Can you work these out from the model? Positions are in its coordinate system, mm. A direction names the side the tool comes from. Coordinates: 2 decimals unless noted, no trailing zeros. Loops run counter-clockwise (first coordinate to the right, second up) from the corner with the lowest first, then second, coordinate; pieces in that order, holes last.
```python
from build123d import *
from build123d import SkipClean  # not in build123d's __all__

# Parameters (mm, degrees)
F1_DEPTH = 4
F2_DEPTH = 2


with BuildPart() as f1:
    # F0 (on Top) → F1 (new body)
    with BuildSketch(Plane.XY):
        Polygon((0, -51.35), (-3.5355339059, -54.8855339059), (54.8855339059, -54.8855339059), (51.35, -51.35), (48.35, -51.35), (44.35, -51.35), (7, -51.35), (3, -51.35), align=None)
        Polygon((7, -7), (0, -7), (0, -44.35), (7, -44.35), (7, -41.3499993608), (7, -10), align=None)
        Polygon((10.0000006392, -44.35), (7, -44.35), (7, -51.35), (44.35, -51.35), (44.35, -44.35), (41.35, -44.35), align=None)
        with BuildLine():
            Line((7, -44.35), (0, -44.35))
            Line((0, -44.35), (0, -48.35))
            Line((0, -48.35), (1.5, -48.35))
            ThreePointArc((1.5, -48.35), (3, -46.85), (4.5, -48.35))
            ThreePointArc((4.5, -48.35), (4.0606601718, -49.4106601718), (3, -49.85))
            Line((3, -49.85), (3, -51.35))
            Line((3, -51.35), (7, -51.35))
            Line((7, -51.35), (7, -44.35))
        make_face()
        with BuildLine():
            Line((0, -48.35), (0, -51.35))
            Line((0, -51.35), (3, -51.35))
            Line((3, -51.35), (3, -49.85))
            ThreePointArc((3, -49.85), (1.9393398282, -49.4106601718), (1.5, -48.35))
            Line((1.5, -48.35), (0, -48.35))
        make_face()
        Polygon((0, -3), (0, 0), (-3.5355339059, 3.5355339059), (-3.5355339059, -54.8855339059), (0, -51.35), (0, -48.35), (0, -44.35), (0, -7), align=None)
        with BuildLine():
            Line((7, 0), (3, 0))
            Line((3, 0), (3, -1.5))
            ThreePointArc((3, -1.5), (4.0606601718, -1.9393398282), (4.5, -3))
            ThreePointArc((4.5, -3), (3, -4.5), (1.5, -3))
            Line((1.5, -3), (0, -3))
            Line((0, -3), (0, -7))
            Line((0, -7), (7, -7))
            Line((7, -7), (7, 0))
        make_face()
        with BuildLine():
            Line((3, 0), (0, 0))
            Line((0, 0), (1.9393398282, -1.9393398282))
            ThreePointArc((1.9393398282, -1.9393398282), (2.4259748515, -1.6141807012), (3, -1.5))
            Line((3, -1.5), (3, 0))
        make_face()
        with BuildLine():
            Line((1.9393398282, -1.9393398282), (0, 0))
            Line((0, 0), (0, -3))
            Line((0, -3), (1.5, -3))
            ThreePointArc((1.5, -3), (1.6141807012, -2.4259748515), (1.9393398282, -1.9393398282))
        make_face()
        Polygon((-3.5355339059, 3.5355339059), (0, 0), (3, 0), (7, 0), (44.35, 0), (48.35, 0), (51.35, 0), (54.8855339059, 3.5355339059), align=None)
        Polygon((44.35, 0), (7, 0), (7, -7), (10, -7), (41.3499993608, -7), (44.35, -7), align=None)
        with BuildLine():
            Line((48.35, 0), (44.35, 0))
            Line((44.35, 0), (44.35, -7))
            Line((44.35, -7), (51.35, -7))
            Line((51.35, -7), (51.35, -3))
            Line((51.35, -3), (49.85, -3))
            ThreePointArc((49.85, -3), (47.2893398282, -4.0606601718), (48.35, -1.5))
            Line((48.35, -1.5), (48.35, 0))
        make_face()
        with BuildLine():
            Line((51.35, -3), (51.35, 0))
            Line((51.35, 0), (48.35, 0))
            Line((48.35, 0), (48.35, -1.5))
            ThreePointArc((48.35, -1.5), (49.4106601718, -1.9393398282), (49.85, -3))
            Line((49.85, -3), (51.35, -3))
        make_face()
        Polygon((54.8855339059, -54.8855339059), (54.8855339059, 3.5355339059), (51.35, 0), (51.35, -3), (51.35, -7), (51.35, -44.35), (51.35, -48.35), (51.35, -51.35), align=None)
        Polygon((51.35, -7), (44.35, -7), (44.35, -10.0000006392), (44.35, -41.35), (44.35, -44.35), (51.35, -44.35), align=None)
        with BuildLine():
            Line((48.35, -51.35), (51.35, -51.35))
            Line((51.35, -51.35), (51.35, -48.35))
            Line((51.35, -48.35), (49.85, -48.35))
            ThreePointArc((49.85, -48.35), (49.4106601718, -49.4106601718), (48.35, -49.85))
            Line((48.35, -49.85), (48.35, -51.35))
        make_face()
        with BuildLine():
            Line((44.35, -51.35), (48.35, -51.35))
            Line((48.35, -51.35), (48.35, -49.85))
            ThreePointArc((48.35, -49.85), (47.2893398282, -47.2893398282), (49.85, -48.35))
            Line((49.85, -48.35), (51.35, -48.35))
            Line((51.35, -48.35), (51.35, -44.35))
            Line((51.35, -44.35), (44.35, -44.35))
            Line((44.35, -44.35), (44.35, -51.35))
        make_face()
        Polygon((7, -41.3499993608), (7, -44.35), (8.5000003196, -42.8499996804), align=None)
        Polygon((8.5000003196, -42.8499996804), (7, -44.35), (10.0000006392, -44.35), align=None)
        Polygon((8.5000003196, -42.8499996804), (10.0000006392, -44.35), (25.6750003196, -28.6750003196), (24.175, -27.175), align=None)
        Polygon((22.6749996804, -25.6749996804), (7, -41.3499993608), (8.5000003196, -42.8499996804), (24.175, -27.175), align=None)
        Polygon((8.5, -8.5), (7, -10), (22.6749996804, -25.6749996804), (24.1749996804, -24.1749996804), align=None)
        Polygon((25.6749996804, -22.6749996804), (10, -7), (8.5, -8.5), (24.1749996804, -24.1749996804), align=None)
        Polygon((27.175, -24.175), (25.6749996804, -22.6749996804), (24.1749996804, -24.1749996804), (25.675, -25.675), align=None)
        Polygon((27.1750003196, -27.1750003196), (28.6750003196, -25.6750003196), (27.175, -24.175), (25.675, -25.675), align=None)
        Polygon((25.675, -25.675), (24.175, -27.175), (25.6750003196, -28.6750003196), (27.1750003196, -27.1750003196), align=None)
        Polygon((24.1749996804, -24.1749996804), (22.6749996804, -25.6749996804), (24.175, -27.175), (25.675, -25.675), align=None)
        Polygon((25.6750003196, -28.6750003196), (41.35, -44.35), (42.85, -42.85), (27.1750003196, -27.1750003196), align=None)
        Polygon((42.85, -42.85), (44.35, -41.35), (28.6750003196, -25.6750003196), (27.1750003196, -27.1750003196), align=None)
        Polygon((8.5, -8.5), (7, -7), (7, -10), align=None)
        Polygon((10, -7), (7, -7), (8.5, -8.5), align=None)
        Polygon((28.6750003196, -25.6750003196), (44.35, -10.0000006392), (42.8499996804, -8.5000003196), (27.175, -24.175), align=None)
        Polygon((42.8499996804, -8.5000003196), (41.3499993608, -7), (25.6749996804, -22.6749996804), (27.175, -24.175), align=None)
        Polygon((44.35, -10.0000006392), (44.35, -7), (42.8499996804, -8.5000003196), align=None)
        Polygon((44.35, -44.35), (44.35, -41.35), (42.85, -42.85), align=None)
        Polygon((42.85, -42.85), (41.35, -44.35), (44.35, -44.35), align=None)
        Polygon((42.8499996804, -8.5000003196), (44.35, -7), (41.3499993608, -7), align=None)
    extrude(amount=F1_DEPTH)

    # F0 (on Top) → F2 (join)
    with BuildSketch(Plane.XY):
        with BuildLine():
            Line((7, -44.35), (0, -44.35))
            Line((0, -44.35), (0, -48.35))
            Line((0, -48.35), (1.5, -48.35))
            ThreePointArc((1.5, -48.35), (3, -46.85), (4.5, -48.35))
            ThreePointArc((4.5, -48.35), (4.0606601718, -49.4106601718), (3, -49.85))
            Line((3, -49.85), (3, -51.35))
            Line((3, -51.35), (7, -51.35))
            Line((7, -51.35), (7, -44.35))
        make_face()
        with BuildLine():
            Line((0, -48.35), (0, -51.35))
            Line((0, -51.35), (3, -51.35))
            Line((3, -51.35), (3, -49.85))
            ThreePointArc((3, -49.85), (1.9393398282, -49.4106601718), (1.5, -48.35))
            Line((1.5, -48.35), (0, -48.35))
        make_face()
        with BuildLine():
            Line((44.35, -51.35), (48.35, -51.35))
            Line((48.35, -51.35), (48.35, -49.85))
            ThreePointArc((48.35, -49.85), (47.2893398282, -47.2893398282), (49.85, -48.35))
            Line((49.85, -48.35), (51.35, -48.35))
            Line((51.35, -48.35), (51.35, -44.35))
            Line((51.35, -44.35), (44.35, -44.35))
            Line((44.35, -44.35), (44.35, -51.35))
        make_face()
        with BuildLine():
            Line((48.35, -51.35), (51.35, -51.35))
            Line((51.35, -51.35), (51.35, -48.35))
            Line((51.35, -48.35), (49.85, -48.35))
            ThreePointArc((49.85, -48.35), (49.4106601718, -49.4106601718), (48.35, -49.85))
            Line((48.35, -49.85), (48.35, -51.35))
        make_face()
        with BuildLine():
            Line((48.35, 0), (44.35, 0))
            Line((44.35, 0), (44.35, -7))
            Line((44.35, -7), (51.35, -7))
            Line((51.35, -7), (51.35, -3))
            Line((51.35, -3), (49.85, -3))
            ThreePointArc((49.85, -3), (47.2893398282, -4.0606601718), (48.35, -1.5))
            Line((48.35, -1.5), (48.35, 0))
        make_face()
        with BuildLine():
            Line((51.35, -3), (51.35, 0))
            Line((51.35, 0), (48.35, 0))
            Line((48.35, 0), (48.35, -1.5))
            ThreePointArc((48.35, -1.5), (49.4106601718, -1.9393398282), (49.85, -3))
            Line((49.85, -3), (51.35, -3))
        make_face()
        with BuildLine():
            Line((7, 0), (3, 0))
            Line((3, 0), (3, -1.5))
            ThreePointArc((3, -1.5), (4.0606601718, -1.9393398282), (4.5, -3))
            ThreePointArc((4.5, -3), (3, -4.5), (1.5, -3))
            Line((1.5, -3), (0, -3))
            Line((0, -3), (0, -7))
            Line((0, -7), (7, -7))
            Line((7, -7), (7, 0))
        make_face()
        with BuildLine():
            Line((1.9393398282, -1.9393398282), (0, 0))
            Line((0, 0), (0, -3))
            Line((0, -3), (1.5, -3))
            ThreePointArc((1.5, -3), (1.6141807012, -2.4259748515), (1.9393398282, -1.9393398282))
        make_face()
        with BuildLine():
            Line((3, 0), (0, 0))
            Line((0, 0), (1.9393398282, -1.9393398282))
            ThreePointArc((1.9393398282, -1.9393398282), (2.4259748515, -1.6141807012), (3, -1.5))
            Line((3, -1.5), (3, 0))
        make_face()
    with SkipClean():  # cleaning this boolean's faces spoils the solid; the shape is the same uncleaned
        extrude(amount=-F2_DEPTH)


solid = f1.part
```
(1) I want a section at D-D on y = -37.5. Write out the boundary of the cut face in (x, z).
Check values:
outline: (-3.54, 0) - (7, 0) - (7, 4) - (-3.54, 4) - close; (10.85, 0) - (16.85, 0) - (16.85, 4) - (10.85, 4) - close; (34.5, 0) - (40.5, 0) - (40.5, 4) - (34.5, 4) - close; (44.35, 0) - (54.89, 0) - (54.89, 4) - (44.35, 4) - close
(2) If we mould it in two halves opening along X, with no side actions, what happens to faces 5 (the flat face through (0, -3, -1)), 6 (the flat face through (7, -48, -1)), 7 (the flat face through (26, -44.35, 2)), 8 (the flat face through (51.35, -48, -1))? For each: released by +X, released by -X, zero draft, split by the parting line, or undercut.
Check values:
face 5: released by -X
face 6: undercut
face 7: undercut
face 8: released by +X
(3) If I drill on probe 1 along X at (y, z) = (-3, 2.5); probe 2 along Y at (x, z) = (48.35, -1); probe 3 along X at (y, z) = (-3, -0.95), over which ranges is the centre line in solid material (lowest first)?
Check values:
probe 1: x = -3.54 to 1.5, 4.5 to 46.85, 49.85 to 54.89
probe 2: y = -51.35 to -49.85, -46.85 to -44.35, -7 to -4.5, -1.5 to 0
probe 3: x = 0 to 1.5, 4.5 to 7, 44.35 to 46.85, 49.85 to 51.35
(4) I want a section at A-A on z = -0.7. Write out the boundary of the cut face in (x, y).
Check values:
outline: (0, -51.35) - (7, -51.35) - (7, -44.35) - (0, -44.35) - close; (0, -7) - (7, -7) - (7, 0) - (0, 0) - close; (44.35, -51.35) - (51.35, -51.35) - (51.35, -44.35) - (44.35, -44.35) - close; (44.35, -7) - (51.35, -7) - (51.35, 0) - (44.35, 0) - close; hole circle Ø3 at (3, -48.35); hole circle Ø3 at (3, -3); hole circle Ø3 at (48.35, -48.35); hole circle Ø3 at (48.35, -3)
(5) I want a section at B-B on y = -8.5. Write out the boundary of the cut face in (x, z), then the cut area to 3 significant figures.
Check values:
outline: (-3.54, 0) - (11.5, 0) - (11.5, 4) - (-3.54, 4) - close; (39.85, 0) - (54.89, 0) - (54.89, 4) - (39.85, 4) - close
area: 120 mm2
(6) I want a section at C-C on x = 31.5. Write out the boundary of the cut face in (y, z).
Check values:
outline: (-54.89, 0) - (-44.35, 0) - (-44.35, 4) - (-54.89, 4) - close; (-34.5, 0) - (-28.5, 0) - (-28.5, 4) - (-34.5, 4) - close; (-22.85, 0) - (-16.85, 0) - (-16.85, 4) - (-22.85, 4) - close; (-7, 0) - (3.54, 0) - (3.54, 4) - (-7, 4) - close
(7) I'm going to push flat-ended pins straight in: pin 1 (4 mm diameter, centred on x = 16, y = -18.5, fed in from -Z); pin 2 (1 mm diameter, centred on x = 47.5, z = -1, fed in from -Y); pin 3 (0.6 mm diameter, centred on y = -4, z = -0.5, fed in from -X); pin 4 (2.5 mm diameter, centred on x = 48.35, y = -48.35, fed in from -Z). Where does each tip first touch, or does it pass through?
Check values:
pin 1: stops at z = 0
pin 2: stops at y = -51.35
pin 3: stops at x = 0
pin 4: passes through
(8) Which directions (+Z, -Z, +X, -X, +Y, -Y) give clear straight access to the entire face, cutting with the end or side of a thin tool? Please do faces 1 (the flat face through (0, -48, -1)), 2 (the flat face through (4, 0, -1)), 3 (the flat face through (4, -44.35, -1)), 4 (the flat face through (37, -34, 2)).
Check values:
face 1: -Z, -X, +Y, -Y
face 2: -Z, +X, -X, +Y
face 3: -Z, +X, -X
face 4: +Z, -Z
